Answer from the drawing. Dimensions are ordinates in mm from the lowest x, y and z of the part. A direction names the side the tool comes from. Coordinates: 2 decimals unless noted, no trailing zeros. Write each loop counter-clockwise with the first axis right and the second up, starting at its lowest first coordinate (ties: lowest second). Pieces come first, ordered by that corner, then holes. Notation, with made-up numbers: (63.25, 45) -> (81.25, 45) arc R16 ccw to (81.25, 73) -> close; hole circle Ø6 at (3, 59.25). An arc over 180 degrees is marked (long way). One line per item, written item: value. Start each with the question number.
1. Given P1, Ø2, axis at y = 6.5, z = 71, coming from the +X side; P2, Ø8, axis at x = 23, z = 69, coming from the +Y side; P3, Ø8, axis at x = 59, y = 22.5, coming from the +Z side, each flat-ended and moving along its own axis, determine where each tip first touches the part or whether it passes through.
2. Find section C-C, the plane x = 47. Write down the section's boundary in (y, z).
3. Find section A-A, the plane y = 3.5. Write down the section's boundary in (x, z) (1 decimal), and give its area (3 significant figures).
4. Find section B-B, the plane z = 8. Write down the section's boundary in (x, y).
5. For the marked faces 1 and 2, determine the directions among +Z, -Z, +X, -X, +Y, -Y from which every point of the face is accessible in a straight line to the end or side of a thin tool.
6. Consider line 1 along Y through (x, z) = (97, 58); line 2 along Z through (x, y) = (23.5, 25.5). Determine where each line is inside the solid, lowest interval first.
7. Find section D-D, the plane y = 22.5. Write down the section's boundary in (x, z).
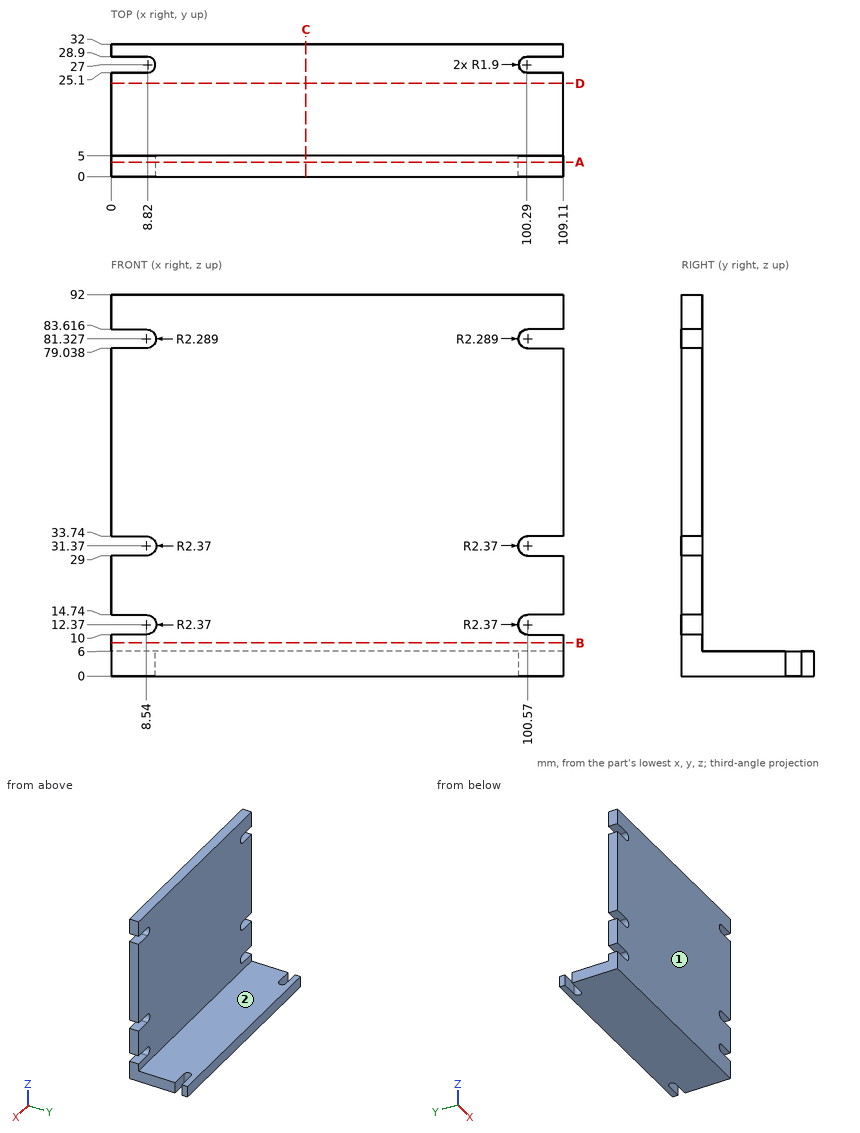
Answer block:
1. P1: passes through
1. P2: stops at y = 5
1. P3: stops at z = 6
2. outline: (0, 0) -> (32, 0) -> (32, 6) -> (5, 6) -> (5, 92) -> (0, 92) -> close
3. outline: (0, 0) -> (109.1, 0) -> (109.1, 10) -> (100.6, 10) arc R2.4 cw to (100.6, 14.7) -> (109.1, 14.7) -> (109.1, 29) -> (100.6, 29) arc R2.4 cw to (100.6, 33.7) -> (109.1, 33.7) -> (109.1, 79) -> (100.6, 79) arc R2.3 cw to (100.6, 83.6) -> (109.1, 83.6) -> (109.1, 92) -> (0, 92) -> (0, 83.6) -> (8.5, 83.6) arc R2.3 cw to (8.5, 79) -> (0, 79) -> (0, 33.7) -> (8.5, 33.7) arc R2.4 cw to (8.5, 29) -> (0, 29) -> (0, 14.7) -> (8.5, 14.7) arc R2.4 cw to (8.5, 10) -> (0, 10) -> close
3. area: 9,750 mm2
4. outline: (0, 0) -> (109.11, 0) -> (109.11, 5) -> (0, 5) -> close
5. face 1: +Z, -Z, +X, -X, -Y
5. face 2: +Z, +X, -X, +Y
6. line 1: y = 0 to 5
6. line 2: z = 0 to 6
7. outline: (0, 0) -> (109.11, 0) -> (109.11, 6) -> (0, 6) -> close
